Autodesk Inventor part; units mm, degrees
ref_plane "YZ Plane" through (0, 0, 0) normal (1, 0, 0) x (0, 1, 0)
ref_plane "XZ Plane" through (0, 0, 0) normal (0, 1, 0) x (-1, 0, 0)
ref_plane "XY Plane" through (0, 0, 0) normal (0, 0, 1) x (1, 0, 0)
sketch "Sketch1" plane through (0, 0, 0) normal (0, 1, 0) x (-1, 0, 0)
  line L0 (53.9548, -48.6252) -> (-46.0452, -48.6252)
  line L1 (-46.0452, -48.6252) -> (-46.0452, -128.6252)
  line L2 (-46.0452, -128.6252) -> (53.9548, -128.6252)
  line L3 (53.9548, -128.6252) -> (53.9548, -48.6252)
  point P0 (0, 0)
  dimension "d6" = 100
  dimension "d7" = 80
extrude "Extrusion1" add sketch "Sketch1" along normal blind 12.7
shell "Shell1" thickness 2.54 removed faces 1 at (12.7119, 12.7, -75.2919)
fillet "Fillet1" radius 2 1 edges at (-3.9548, 12.7, -128.6252)
sketch "Sketch2" plane through (-51.4148, 2.54, -126.0852) normal (0, 1, 0) x (1, 0, 0)
  circle A0 centre (11.4204, -24.6498) radius 2.5
  point P0 (51.4148, -126.0852)
  dimension "d8" = 5
extrude "Extrusion2" cut sketch "Sketch2" against normal blind 10
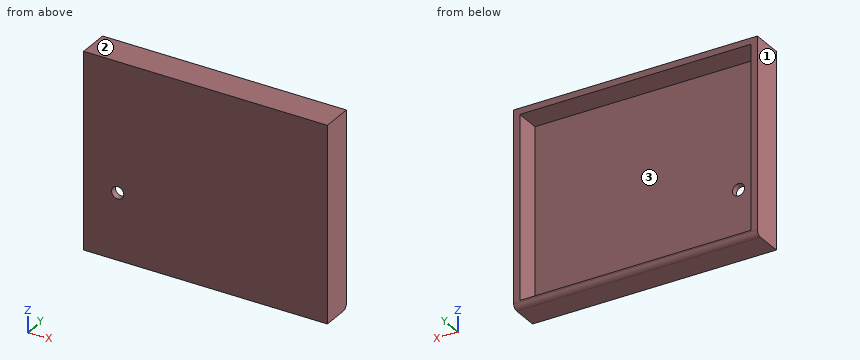
The model under review builds one solid part; all positions refer to its coordinate system, in mm. Face numbers are marked on the shaded views. Round coordinates to 2 decimals unless told otherwise and drop trailing zeros. Write each loop counter-clockwise with the first axis right and the second up, starting at its lowest first coordinate (ties: lowest second). Pieces come first, ordered by that corner, then holes. Notation, with made-up numbers: M -13,89.5 L 27,89.5 A18 cw 27,111.5 Z; hole C 39.25,87 d6. An arc over 180 degrees is marked long. Answer as CSV lines item,"result". Start each with the question number.
Q1. Consider section B-B, the plane x = -30. Give the boundary of the cut face in (y, z), then the cut area to 3 significant figures.
Q2. Consider section A-A, the plane y = 7.75. Give the boundary of the cut face in (x, z), then the cut area to 3 significant figures.
Q3. Wall thickness on line 1 along Z through (x, y) = (-26, 6); line 2 along X through (y, z) = (7.25, -116); line 3 along Y through (x, z) = (-34, -122): over which ranges is each line inside the solid? List them lowest first.
Q4. Clearance check with a flat-ended pin moving along its axis: P1, Ø4, axis at x = -43.5, z = -105, coming from the +Y side. State where the tip first meets the part, or that it passes through.
Q5. The part is to be moulded in two halves that separate along X. For the marked faces 1, 2 and 3, say which applies: +X half, -X half, draft (parallel to the pull), parting line (faces both ways), or undercut.
Q6. Consider section C-C, the plane z = -53.5. Give the boundary of the cut face in (x, y), then the cut area to 3 significant figures.
Result set:
1,outline,"M 0,-128.63 L 10.7,-128.63 A2 ccw 12.7,-126.63 L 12.7,-126.09 L 2.54,-126.09 L 2.54,-51.17 L 12.7,-51.17 L 12.7,-48.63 L 0,-48.63 Z"
1,area,"254 mm²"
2,outline,"M -53.95,-128.63 L 46.05,-128.63 L 46.05,-48.63 L -53.95,-48.63 Z; hole M -51.41,-126.09 L 43.51,-126.09 L 43.51,-51.17 L -51.41,-51.17 Z"
2,area,"889 mm²"
3,line 1,"z = -128.63 to -126.09, -51.17 to -48.63"
3,line 2,"x = -53.95 to -51.41, 43.51 to 46.05"
3,line 3,"y = 0 to 2.54"
4,P1,"stops at y = 2.54"
5,face 1,"-X half"
5,face 2,"draft"
5,face 3,"undercut"
6,outline,"M -53.95,0 L 46.05,0 L 46.05,12.7 L 43.51,12.7 L 43.51,2.54 L -51.41,2.54 L -51.41,12.7 L -53.95,12.7 Z"
6,area,"306 mm²"
